```python
from build123d import *

# Parameters (mm, degrees)
SKETCH1_W                = 203.2
SKETCH1_H                = 50.8
SKETCH1_R                = 6.25
SKETCH1_R_2              = 3.175
BOSS_EXTRUDE1_DEPTH      = 6.35
SKETCH2_W                = 41.159999976
SKETCH2_H                = 3.175
CUT_EXTRUDE1_DEPTH       = 3.175
SKETCH3_W                = 4.7625
SKETCH3_H                = 50.8
CUT_EXTRUDE2_DEPTH       = 3.175
SKETCH4_R                = 4.7625
CUT_EXTRUDE3_DEPTH       = 105.919218926
BOSS_EXTRUDE2_DEPTH      = 6.35
BOSS_EXTRUDE2_DEPTH_BACK = 57.15
SKETCH5_W                = 41.159999976
SKETCH5_H                = 3.175
SKETCH6_R                = 1.5
CUT_EXTRUDE4_DEPTH       = 6.35


with BuildPart() as part:
    # Sketch1 → Boss-Extrude1 (new body)
    with BuildSketch(Plane(origin=(0, 0, 0), x_dir=(1, 0, 0), z_dir=(0, 1, 0))):
        Rectangle(SKETCH1_W, SKETCH1_H)
        with Locations(Location((-82.55, 0, 0), (0, 0, 270))):
            Circle(SKETCH1_R, mode=Mode.SUBTRACT)
        with Locations(Location((82.55, 0, 0), (0, 0, 90))):
            Circle(SKETCH1_R, mode=Mode.SUBTRACT)
        with Locations(Location((0, 0, 0), (0, 0, 270))):
            Circle(SKETCH1_R_2, mode=Mode.SUBTRACT)
    extrude(amount=BOSS_EXTRUDE1_DEPTH)

    # Sketch2 → Cut-Extrude1 (cut)
    with BuildSketch(Plane(origin=(0, 6.35, 0), x_dir=(1, 0, 0), z_dir=(0, 1, 0))):
        with Locations((0, -23.8125)):
            Rectangle(SKETCH2_W, SKETCH2_H)
        with Locations((0, 23.8125)):
            Rectangle(SKETCH2_W, SKETCH2_H)
    extrude(amount=-CUT_EXTRUDE1_DEPTH, mode=Mode.SUBTRACT)

    # Sketch3 → Cut-Extrude2 (cut)
    with BuildSketch(Plane.XZ):
        with Locations((-99.21875, 0)):
            Rectangle(SKETCH3_W, SKETCH3_H)
        with Locations((99.21875, 0)):
            Rectangle(SKETCH3_W, SKETCH3_H)
    extrude(amount=-CUT_EXTRUDE2_DEPTH, mode=Mode.SUBTRACT)

    # Sketch4 → Cut-Extrude3 (cut, through all)
    with BuildSketch(Plane(origin=(0, 6.35, 0), x_dir=(1, 0, 0), z_dir=(0, 1, 0))):
        with Locations(Location((-26.035, 0, 0), (0, 0, 270))):
            Circle(SKETCH4_R)
        with Locations(Location((26.035, 0, 0), (0, 0, 90))):
            Circle(SKETCH4_R)
    extrude(amount=-CUT_EXTRUDE3_DEPTH, mode=Mode.SUBTRACT)

    # Sketch5 → Boss-Extrude2 (add, two sides: drawn at the far end of the back side and taken through both)
    with BuildSketch(Plane(origin=(0, 0, -25.4), x_dir=(-1, 0, 0), z_dir=(0, 0, -1)).offset(-BOSS_EXTRUDE2_DEPTH_BACK)):
        with Locations((0, 1.5875)):
            Rectangle(SKETCH5_W, SKETCH5_H)
    extrude(amount=BOSS_EXTRUDE2_DEPTH + BOSS_EXTRUDE2_DEPTH_BACK)

    # Sketch6 → Cut-Extrude4 (cut)
    with BuildSketch(Plane(origin=(0, 3.175, 0), x_dir=(1, 0, 0), z_dir=(0, 1, 0))):
        with Locations(Location((-14.229999988, 28.575, 0), (0, 0, 270))):
            Circle(SKETCH6_R)
        with Locations(Location((14.229999988, 28.575, 0), (0, 0, 90))):
            Circle(SKETCH6_R)
        with Locations(Location((14.229999988, -28.575, 0), (0, 0, 270))):
            Circle(SKETCH6_R)
        with Locations(Location((-14.229999988, -28.575, 0), (0, 0, 90))):
            Circle(SKETCH6_R)
    extrude(amount=-CUT_EXTRUDE4_DEPTH, mode=Mode.SUBTRACT)


solid = part.part
```
Here's how the part is built. I have some questions about the finished solid (model axes, mm). A direction names the side the tool comes from. Coordinates: 2 decimals unless noted, no trailing zeros. Write each loop counter-clockwise with the first axis right and the second up, starting at its lowest first coordinate (ties: lowest second). Pieces come first, ordered by that corner, then holes. Notation, with made-up numbers: (72, 87) -> (106, 87) arc R30 cw to (106, 112) -> close; hole circle Ø4 at (-23, 42). An arc over 180 degrees is marked (long way). Use a Markdown table: item, result. Add a question column.
(1) Please list where these lines run through material, in increasing order: line 1 (X direction, y = 1.25, z = 0); line 2 (X direction, y = 5.6, z = 0) (1 decimal); line 3 (X direction, y = 5.75, z = 1).
(2) I'm going to push flat-ended pins straight in: P1, Ø1.9, axis at x = 78.5, y = 2.5, coming from the -Z side; P2, Ø1, axis at y = 1, z = 10, coming from the +X side; P3, Ø7.5, axis at x = 82.55, z = 0, coming from the -Y side; P4, Ø15, axis at x = 26.035, z = 0, coming from the +Y side. Where does each tip first touch, or does it pass through?
(3) For faces 1 (the flat face through (-62, 3, -25.4)), 2 (the flat face through (-62, 3, 25.4)), 3 (the cylindrical face through (-1.93, 4.74, -2.52)), 4 (the flat face through (99, 3.175, 0)), which set-ups out of +Z, -Z, +X, -X, +Y, -Y let a thin tool reach every point of the face, with its end or its side?
(4) If we section it at D-D, the plane x = 43.5: Write out the boundary of the cut face in (y, z), and give its area (3 significant figures).
(5) If we section it at A-A, the plane z = 0: State how many separate pieces and enclosed holes the cut face has, and give its area (3 significant figures).
(6) We'd pull the mould along X, two halves only. Please class faces 5 (the flat face through (0, 3.175, 0)), 6 (the flat face through (61, 3, 25.4)): +X half, -X half, draft (parallel to the pull), parting line (faces both ways), or undercut.
(7) If we section it at B-B, the plane x = -82.55: Write out the boundary of the cut face in (y, z), and give its area (3 significant figures).
Outcome:
| question | item | result |
|---|---|---|
| 1 | line 1 | x = -96.84 to -88.8, -76.3 to -30.8, -21.27 to 21.27, 30.8 to 76.3, 88.8 to 96.84 |
| 1 | line 2 | x = -101.6 to -88.8, -76.3 to -30.8, -21.3 to -3.2, 3.2 to 21.3, 30.8 to 76.3, 88.8 to 101.6 |
| 1 | line 3 | x = -101.6 to -88.72, -76.38 to -30.69, -21.38 to -3.01, 3.01 to 21.38, 30.69 to 76.38, 88.72 to 101.6 |
| 2 | P1 | stops at z = -25.4 |
| 2 | P2 | stops at x = 96.84 |
| 2 | P3 | passes through |
| 2 | P4 | stops at y = 6.35 |
| 3 | face 1 | -Z, -X, +Y, -Y |
| 3 | face 2 | +Z, -X, +Y, -Y |
| 3 | face 3 | +Y |
| 3 | face 4 | +Z, -Z, +X, -Y |
| 4 | outline | (0, -25.4) -> (6.35, -25.4) -> (6.35, 25.4) -> (0, 25.4) -> close |
| 4 | area | 323 mm^2 |
| 5 | separate pieces | 5 |
| 5 | enclosed holes | 0 |
| 5 | area | 960 mm^2 |
| 6 | face 5 | undercut |
| 6 | face 6 | draft |
| 7 | outline | (0, -25.4) -> (6.35, -25.4) -> (6.35, -6.25) -> (0, -6.25) -> close; (0, 6.25) -> (6.35, 6.25) -> (6.35, 25.4) -> (0, 25.4) -> close |
| 7 | area | 243 mm^2 |
